Design review of the part built by this model. Coordinates are the model's own, in mm. Face numbers are marked on the shaded views. A direction names the side the tool comes from. Round coordinates to 2 decimals unless told otherwise and drop trailing zeros. Order: outer loops, then holes, each group sorted by start corner. A loop starts at its lowest first (then second) coordinate and runs counter-clockwise, first axis right, second up. Notation, with made-up numbers: M -25.5,42 L -0.5,42 A18 cw -0.5,66 Z; hole C 53,62 d3. An arc over 180 degrees is marked long. Write each question's results on one line, items separated by ' | '. Start each with the question number.
Item 1: Take a section at A-A, the plane x = 0. Write out the cut boundary in (y, z), plus the area to 3 significant figures.
Item 2: Take a section at C-C, the plane y = -1. Write out the cut boundary in (x, z), plus the area to 3 significant figures.
Item 3: Machinability: for the marked faces 4, 5, 6 and 7, which of the approach directions +Z, -Z, +X, -X, +Y, -Y give a long, thin tool a straight path to every point of the face, cutting with its end or side? Answer none if there is none.
Item 4: The part is to be moulded in two halves that separate along X. For the marked faces 1, 2 and 3, say which applies: +X half, -X half, draft (parallel to the pull), parting line (faces both ways), or undercut.
Item 5: Take a section at B-B, the plane z = -20. Write out the cut boundary in (x, y).
Item 6: Take a section at D-D, the plane y = 29.5. Write out the cut boundary in (x, z).
Item 7: Wall thickness on line 1 (Z direction, x = -0.5, y = 6); line 2 (X direction, y = 27, z = 1); line 3 (Y direction, x = -5, z = -14): over which ranges is each line inside the solid? List them lowest first. Write a range as [from, to].
Item 8: Clearance check with flat-ended pins moving along their axes: pin 1 (5 mm diameter, centred on y = 5.5, z = -17, fed in from +X); pin 2 (1.6 mm diameter, centred on x = -7, y = -10.5, fed in from -Z); pin 3 (13 mm diameter, centred on x = 6.5, z = -0.5, fed in from -Y). State where each tip first meets the part, or that it passes through.
```python
from build123d import *
from OCP.BRepFilletAPI import BRepFilletAPI_MakeChamfer

# Parameters (mm, degrees)
BOSS_EXTRUDE1_DEPTH     = 12
SKETCH2_W               = 8
SKETCH2_H               = 12
BOSS_EXTRUDE2_DEPTH     = 14.74
CUT_EXTRUDE1_DEPTH      = 37.164969238
CUT_EXTRUDE1_DEPTH_BACK = 37.164969238
SKETCH3_W               = 14.74
SKETCH3_H               = 1.25
CUT_EXTRUDE2_DEPTH      = 37.164969238
CUT_EXTRUDE2_DEPTH_BACK = 37.164969238
SKETCH4_R               = 3.55
CUT_EXTRUDE3_DEPTH      = 37.164969238
CUT_EXTRUDE3_DEPTH_BACK = 37.164969238
SKETCH6_W               = 2
SKETCH6_H               = 10.75
FILLET1_R               = 4
BOSS_EXTRUDE3_DEPTH     = 8
SKETCH8_R               = 13.05
SKETCH8_R_2             = 8.05
BOSS_EXTRUDE4_DEPTH     = 20
SKETCH9_W               = 3.9
SKETCH9_H               = 7.5
BOSS_EXTRUDE5_DEPTH     = 11.9
CUT_EXTRUDE4_DEPTH      = 49.820129045
CUT_EXTRUDE4_DEPTH_BACK = 49.820129045
CHAMFER1_SIZE           = 11.9
CHAMFER1_SIZE_2         = 0.5
FILLET3_R               = 1


with BuildPart() as part:
    # Sketch1 → Boss-Extrude1 (new body)
    with BuildSketch(Plane(origin=(0, 0, 0), x_dir=(1, 0, 0), z_dir=(0, 1, 0))):
        with BuildLine():
            Line((-13.05, 8.5), (-13.05, -27.55))
            ThreePointArc((-13.05, -27.55), (-12.464213562, -28.964213562), (-11.05, -29.55))
            Line((-11.05, -29.55), (11.05, -29.55))
            ThreePointArc((11.05, -29.55), (12.464213562, -28.964213562), (13.05, -27.55))
            Line((13.05, -27.55), (13.05, 8.5))
            ThreePointArc((13.05, 8.5), (12.745947042, 9.827507004), (11.894409938, 10.890337003))
            ThreePointArc((11.894409938, 10.890337003), (10.498447473, 12.632681264), (10, 14.808922253))
            Line((10, 14.808922253), (-10, 14.808922253))
            ThreePointArc((-10, 14.808922253), (-10.498447473, 12.632681264), (-11.894409938, 10.890337003))
            ThreePointArc((-11.894409938, 10.890337003), (-12.745947042, 9.827507004), (-13.05, 8.5))
        make_face()
    extrude(amount=BOSS_EXTRUDE1_DEPTH)

    # Sketch2 → Boss-Extrude2 (add)
    with BuildSketch(Plane(origin=(0, 0, -14.808922253), x_dir=(-1, 0, 0), z_dir=(0, 0, -1))):
        with Locations((0, 6)):
            Rectangle(SKETCH2_W, SKETCH2_H)
    extrude(amount=BOSS_EXTRUDE2_DEPTH)

    # Sketch3 → Cut-Extrude1 (cut, two sides: drawn at the far end of the back side and taken through both)
    with BuildSketch(Plane(origin=(4, 0, 0), x_dir=(0, 0, -1), z_dir=(1, 0, 0)).offset(-CUT_EXTRUDE1_DEPTH_BACK)):
        with Locations((22.178922253, 0.625)):
            Rectangle(SKETCH3_W, SKETCH3_H)
    extrude(amount=CUT_EXTRUDE1_DEPTH + CUT_EXTRUDE1_DEPTH_BACK, mode=Mode.SUBTRACT)

    # Sketch4 → Cut-Extrude2 (cut, two sides: drawn at the far end of the back side and taken through both)
    with BuildSketch(Plane(origin=(4, 0, 0), x_dir=(0, 0, -1), z_dir=(1, 0, 0)).offset(-CUT_EXTRUDE2_DEPTH_BACK)):
        with Locations((22.548922253, 6)):
            Circle(SKETCH4_R)
    extrude(amount=CUT_EXTRUDE2_DEPTH + CUT_EXTRUDE2_DEPTH_BACK, mode=Mode.SUBTRACT)

    # Sketch6 → Cut-Extrude3 (cut, two sides: drawn at the far end of the back side and taken through both)
    with BuildSketch(Plane(origin=(4, 0, 0), x_dir=(0, 0, -1), z_dir=(1, 0, 0)).offset(-CUT_EXTRUDE3_DEPTH_BACK)):
        with Locations((28.548922253, 6.625)):
            Rectangle(SKETCH6_W, SKETCH6_H)
    extrude(amount=CUT_EXTRUDE3_DEPTH + CUT_EXTRUDE3_DEPTH_BACK, mode=Mode.SUBTRACT)

    # Fillet1
    fillet1_edges = [part.edges().sort_by_distance(p)[0] for p in [
        (0, 1.25, -27.548922253),
    ]]
    fillet(fillet1_edges, radius=FILLET1_R)

    # Sketch7 → Boss-Extrude3 (add)
    with BuildSketch(Plane(origin=(4, 0, 0), x_dir=(0, 0, -1), z_dir=(1, 0, 0))):
        with BuildLine():
            Line((27.548922253, 10), (27.548922253, 6))
            ThreePointArc((27.548922253, 6), (27.773781475, 7.398207316), (28.122230045, 8.770843088))
            ThreePointArc((28.122230045, 8.770843088), (28.441674093, 10.200150162), (28.548922253, 11.660787366))
            Line((28.548922253, 11.660787366), (28.548922253, 12))
            Line((28.548922253, 12), (27.548922253, 12))
            Line((27.548922253, 12), (27.548922253, 10))
        make_face()
    extrude(amount=-BOSS_EXTRUDE3_DEPTH)

    # Sketch8 → Boss-Extrude4 (add)
    with BuildSketch(Plane(origin=(0, 12, 0), x_dir=(1, 0, 0), z_dir=(0, 1, 0))):
        with Locations(Location((0, -1.5, 0), (0, 0, 180))):
            Circle(SKETCH8_R)
        with Locations(Location((0, -1.5, 0), (0, 0, 270))):
            Circle(SKETCH8_R_2, mode=Mode.SUBTRACT)
    extrude(amount=BOSS_EXTRUDE4_DEPTH)

    # Sketch9 → Boss-Extrude5 (add)
    with BuildSketch(Plane.XZ):
        with Locations((-7.05, 21.8)):
            Rectangle(SKETCH9_W, SKETCH9_H)
        with Locations((7.05, 21.8)):
            Rectangle(SKETCH9_W, SKETCH9_H)
    extrude(amount=BOSS_EXTRUDE5_DEPTH)

    # Sketch10 → Cut-Extrude4 (cut, two sides: drawn at the far end of the back side and taken through both)
    with BuildSketch(Plane.ZY.offset(9).offset(-CUT_EXTRUDE4_DEPTH_BACK)):
        with BuildLine():
            Line((21.25, -3.49), (13.718722393, -3.49))
            Line((13.718722393, -3.49), (13.718722393, -8.49))
            Line((13.718722393, -8.49), (21.25, -8.49))
            ThreePointArc((21.25, -8.49), (23.75, -5.99), (21.25, -3.49))
        make_face()
    extrude(amount=CUT_EXTRUDE4_DEPTH + CUT_EXTRUDE4_DEPTH_BACK, mode=Mode.SUBTRACT)

    # Chamfer1
    chamfer1_edges_1 = [part.edges().sort_by_distance(p)[0] for p in [
        (-7.05, -11.9, 25.55),
    ]]
    chamfer1_side_1 = [part.faces().sort_by_distance(p)[0] for p in [
        (-7.05, -11.89, 25.55),
    ]]
    chamfer1_edges_2 = [part.edges().sort_by_distance(p)[0] for p in [
        (7.05, -11.9, 25.55),
    ]]
    chamfer1_side_2 = [part.faces().sort_by_distance(p)[0] for p in [
        (7.05, -11.89, 25.55),
    ]]
    chamfer1 = BRepFilletAPI_MakeChamfer(part.part.solid().wrapped)
    for e in chamfer1_edges_1:
        chamfer1.Add(CHAMFER1_SIZE - 0.0001, CHAMFER1_SIZE_2 - 0.0001, e.wrapped, chamfer1_side_1[0].wrapped)
    for e in chamfer1_edges_2:
        chamfer1.Add(CHAMFER1_SIZE - 0.0001, CHAMFER1_SIZE_2 - 0.0001, e.wrapped, chamfer1_side_2[0].wrapped)
    add(Compound.cast(chamfer1.Shape()), mode=Mode.REPLACE)  # a hair under: the kernel refuses the full size

    # Fillet3
    fillet3_edges = [part.edges().sort_by_distance(p)[0] for p in [
        (-7.05, -11.9, 18.05),
        (7.05, -11.9, 18.05),
        (7.05, -8.49, 18.05),
        (-7.05, -8.49, 18.05),
        (7.05, -3.49, 18.05),
        (-7.05, -3.49, 18.05),
        (-7.05, -11.9, 25.0501),
        (7.05, -11.9, 25.0501),
    ]]
    fillet(fillet3_edges, radius=FILLET3_R)


solid = part.part
```
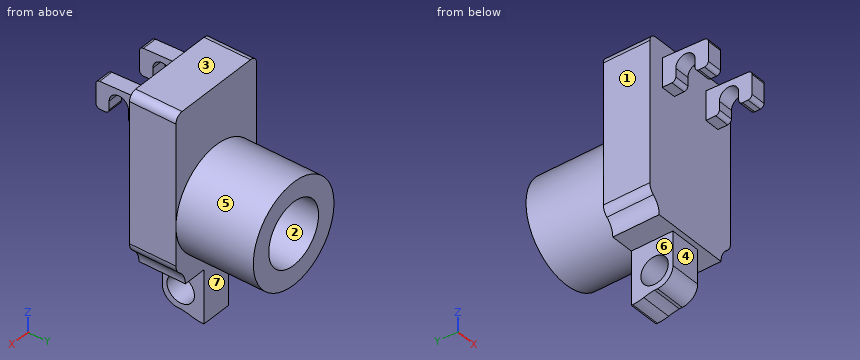
Results list:
1) outline: M 0,-14.81 L 1.25,-14.81 L 1.25,-23.55 A4 ccw 5.25,-27.55 L 6,-27.55 A15.89 cw 8.77,-28.12 A10 ccw 11.66,-28.55 L 12,-28.55 L 12,-11.55 L 32,-11.55 L 32,-6.55 L 12,-6.55 L 12,9.55 L 32,9.55 L 32,14.55 L 12,14.55 L 12,29.55 L 0,29.55 Z; hole C 6,-22.55 d7.1 | area: 830 mm²
2) outline: M -9,18.05 L -5.1,18.05 L -5.1,25.51 L -9,25.51 Z; M 5.1,18.05 L 9,18.05 L 9,25.51 L 5.1,25.51 Z | area: 58.2 mm²
3) face 4: -Z, +X, -X, -Y | face 5: +Y | face 6: -Z, -X, +Y, -Y | face 7: -Z, +Y
4) face 1: -X half | face 2: undercut | face 3: draft
5) outline: M -4,1.25 L 4,1.25 L 4,3.53 L -4,3.53 Z; M -4,8.47 L 4,8.47 L 4,12 L -4,12 Z
6) outline: C 0,1.5 d26.1; hole C 0,1.5 d16.1
7) line 1: [-27.55, -26.1], [-19, 29.55] | line 2: [-13.04, -8.03], [8.03, 13.04] | line 3: [0, 12]
8) pin 1: x = 10.01 | pin 2: z = 18.05 | pin 3: y = 0
